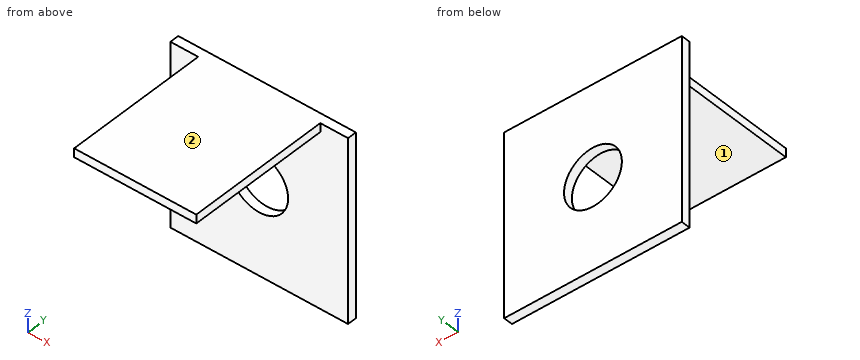
```python
from build123d import *

# Parameters (mm, degrees)
F0_W     = 39
F0_H     = 40
F1_DEPTH = 2
F2_W     = 26.8125
F2_H     = 1.9177
F3_DEPTH = 31.75
F5_D     = 12.7
F5_DEPTH = 76.2


with BuildPart() as f1:
    # F0 (on Front) → F1 (new body)
    with BuildSketch(Plane.XZ):
        with Locations((4.479941, -15.969917)):
            Rectangle(F0_W, F0_H)
    extrude(amount=F1_DEPTH)

    # F2 (on face) → F3 (join)
    with BuildSketch(Plane.XZ.offset(2)):
        with Locations((4.479941, 3.071233)):
            Rectangle(F2_W, F2_H)
    extrude(amount=F3_DEPTH)

    # F5
    with Locations(Plane.XZ.offset(2)):
        with Locations((4.479941, -15.969917)):
            Hole(F5_D / 2, depth=F5_DEPTH)


solid = f1.part
```
The listing builds one solid part. Answer for the finished solid, in the listing's coordinates (mm). Face numbers are marked on the shaded views. A direction names the side the tool comes from. Give positions to 0.01 mm unless a question says otherwise; leave off trailing zeros. Loops run counter-clockwise (first coordinate to the right, second up) from the corner with the lowest first, then second, coordinate; pieces in that order, holes last. Notation, with made-up numbers: M -31,-33.75 L 2,-33.75 A10 cw 2,-28.75 Z; hole C 71,-19.75 d5. An arc over 180 degrees is marked long. One line per item, written item: value.
1. Find the intervals of material crossed by probe 1 along Y at (x, z) = (13, 2); probe 2 along Z at (x, y) = (5, -31); probe 3 along X at (y, z) = (-1.5, -15), in increasing order.
Found:
probe 1: -2 to 0
probe 2: 2.11 to 4.03
probe 3: -15.02 to -1.8, 10.76 to 23.98
2. Each of these flat-tipped pins is pushed along its axis until it touches: P1, Ø5, axis at x = 19, y = -28, coming from the -Z side; P2, Ø5, axis at x = -8, z = -31.5, coming from the -Y side; P3, Ø7.5, axis at x = 4.48, z = -15.97, coming from the -Y side; P4, Ø1, axis at y = -16, z = 3.5, coming from the +X side. Where does it stop, or does it pass through?
Found:
P1: z = 2.11
P2: y = -2
P3: through
P4: x = 17.89
3. Section D-D on y = -25.5 is taken. Determine the outline of the cut face in (x, z).
Found:
outline: M -8.93,2.11 L 17.89,2.11 L 17.89,4.03 L -8.93,4.03 Z
4. Section B-B on x = 0.5 is taken. Determine the outline of the cut face in (y, z).
Found:
outline: M -33.75,2.11 L -2,2.11 L -2,-11.02 L 0,-11.02 L 0,4.03 L -33.75,4.03 Z; M -2,-35.97 L 0,-35.97 L 0,-20.92 L -2,-20.92 Z
5. For the marked faces 1 and 2, determine the directions among +Z, -Z, +X, -X, +Y, -Y from which every point of the face is accessible in a straight line to the end or side of a thin tool.
Found:
face 1: -Z, +X, -X, -Y
face 2: +Z, +X, -X, +Y, -Y
6. Section C-C on x = 12.5 is taken. Determine the outline of the cut face in (y, z).
Found:
outline: M -33.75,2.11 L -2,2.11 L -2,-35.97 L 0,-35.97 L 0,4.03 L -33.75,4.03 Z
7. Section A-A on z = -15 is taken. Determine the outline of the cut face in (x, y).
Found:
outline: M -15.02,-2 L -1.8,-2 L -1.8,0 L -15.02,0 Z; M 10.76,-2 L 23.98,-2 L 23.98,0 L 10.76,0 Z
